from build123d import *

# Parameters (mm, degrees)
SKETCH1_W           = 27.5
SKETCH1_H           = 65
BOSS_EXTRUDE1_DEPTH = 5
SKETCH2_W           = 55
SKETCH2_H           = 130
SKETCH2_W_2         = 45
SKETCH2_H_2         = 120
BOSS_EXTRUDE2_DEPTH = 50.5
SKETCH3_W           = 10
SKETCH3_H           = 10
BOSS_EXTRUDE4_DEPTH = 5
SKETCH4_R           = 2
CUT_EXTRUDE1_DEPTH  = 5
FILLET1_R           = 1
FILLET2_R           = 1
SKETCH6_W           = 38
SKETCH6_H           = 45.3
CUT_EXTRUDE2_DEPTH  = 5
FILLET3_R           = 3
CUT_EXTRUDE3_DEPTH  = 5
FILLET4_R           = 2


with BuildPart() as part:
    # Sketch1 → Boss-Extrude1 (new body)
    with BuildSketch(Plane(origin=(0, 0, 0), x_dir=(1, 0, 0), z_dir=(0, 1, 0))):
        Polygon((27.5, 0), (0, 0), (0, 65), (-27.5, 65), (-27.5, -65), (27.5, -65), align=None)
        with Locations((13.75, 32.5)):
            Rectangle(SKETCH1_W, SKETCH1_H)
    extrude(amount=BOSS_EXTRUDE1_DEPTH)

    # Sketch2 → Boss-Extrude2 (add)
    with BuildSketch(Plane(origin=(0, 5, 0), x_dir=(1, 0, 0), z_dir=(0, 1, 0))):
        Rectangle(SKETCH2_W, SKETCH2_H)
        Rectangle(SKETCH2_W_2, SKETCH2_H_2, mode=Mode.SUBTRACT)
    extrude(amount=BOSS_EXTRUDE2_DEPTH)

    # Sketch3 → Boss-Extrude4 (add)
    with BuildSketch(Plane(origin=(0, 55.5, 0), x_dir=(1, 0, 0), z_dir=(0, 1, 0))):
        with Locations((22.5, 70)):
            Rectangle(SKETCH3_W, SKETCH3_H)
        with Locations((-22.5, -70)):
            Rectangle(SKETCH3_W, SKETCH3_H)
    extrude(amount=-BOSS_EXTRUDE4_DEPTH)

    # Sketch4 → Cut-Extrude1 (cut)
    with BuildSketch(Plane.XZ.offset(-50.5)):
        with Locations(Location((22.5, -70, 0), (0, 0, 270))):
            Circle(SKETCH4_R)
        with Locations(Location((-22.5, 70, 0), (0, 0, 270))):
            Circle(SKETCH4_R)
    extrude(amount=-CUT_EXTRUDE1_DEPTH, mode=Mode.SUBTRACT)

    # Fillet1
    fillet1_edges = [part.edges().sort_by_distance(p)[0] for p in [
        (22.5, 50.5, -68),
    ]]
    fillet(fillet1_edges, radius=FILLET1_R)

    # Fillet2
    fillet2_edges = [part.edges().sort_by_distance(p)[0] for p in [
        (-22.5, 50.5, 72),
    ]]
    fillet(fillet2_edges, radius=FILLET2_R)

    # Sketch6 → Cut-Extrude2 (cut)
    with BuildSketch(Plane.XZ):
        Rectangle(SKETCH6_W, SKETCH6_H)
    extrude(amount=-CUT_EXTRUDE2_DEPTH, mode=Mode.SUBTRACT)

    # Fillet3
    fillet3_edges = [part.edges().sort_by_distance(p)[0] for p in [
        (17.5, 53, -75),
        (27.5, 53, -75),
        (-17.5, 53, 75),
        (-27.5, 53, 75),
    ]]
    fillet(fillet3_edges, radius=FILLET3_R)

    # Sketch8 → Cut-Extrude3 (cut)
    with BuildSketch(Plane(origin=(0, 0, -65), x_dir=(-1, 0, 0), z_dir=(0, 0, -1))):
        Polygon((0, 55.5), (5, 55.5), (5, 45.5), (-5, 45.5), (-5, 55.5), align=None)
    extrude(amount=-CUT_EXTRUDE3_DEPTH, mode=Mode.SUBTRACT)

    # Fillet4
    fillet4_edges = [part.edges().sort_by_distance(p)[0] for p in [
        (-5, 45.5, -62.5),
        (5, 45.5, -62.5),
    ]]
    fillet(fillet4_edges, radius=FILLET4_R)


solid = part.part
The listing builds one solid part. Answer for the finished solid, in the listing's coordinates (mm). A direction names the side the tool comes from. Give positions to 0.01 mm unless a question says otherwise; leave off trailing zeros. Write each loop counter-clockwise with the first axis right and the second up, starting at its lowest first coordinate (ties: lowest second). Pieces come first, ordered by that corner, then holes.
Item 1: Section D-D, the plane z = -4 is taken. Write down the section's boundary in (x, y).
Item 2: Which of the six approach directions +Z, -Z, +X, -X, +Y, -Y give full straight-line access (tool end or side, diameter ignored) to faces 1 (the flat face through (22.5, 30, 1)), 2 (the flat face through (19, 2, 0)), 3 (the flat face through (0, 45.5, -63)), 4 (the flat face through (17.5, 53, -68))?
Item 3: Section C-C, the plane y = 39 is taken. Write down the section's boundary in (x, z), plus the area to 3 significant figures.
Item 4: Section B-B, the plane z = 70 is taken. Write down the section's boundary in (x, y), plus the area to 3 significant figures.
Item 5: Section A-A, the plane x = -14.5 is taken. Write down the section's boundary in (y, z).
Item 6: Flat-ended cylindrical pins translate along their axes: P1, Ø2, axis at x = -2, y = 32.5, coming from the -Z side; P2, Ø4, axis at x = 4, z = -44, coming from the +Y side; P3, Ø1.5, axis at y = 53.5, z = -67.5, coming from the -X side. Find the tip coordinate at first contact, or state that the pin passes through.
Item 7: Find the intervals of material crossed by line 1 along Z through (x, y) = (19, 45); line 2 along X through (y, z) = (54.2, 70); line 3 along Z through (x, y) = (22, 53), in increasing order.
Item 8: Determine the mould class of faces 5 (the cylindrical face through (-18.4, 52.96, 74.14)), 6 (the flat face through (-25, 50.5, 68)), 7 (the flat face through (20, 5, -1)) for opening direction X: released by +X, released by -X, zero draft, split by the parting line, or undercut.
Completed:
1. outline: (-27.5, 0) - (-19, 0) - (-19, 5) - (-22.5, 5) - (-22.5, 55.5) - (-27.5, 55.5) - close; (19, 0) - (27.5, 0) - (27.5, 55.5) - (22.5, 55.5) - (22.5, 5) - (19, 5) - close
2. face 1: +Y
2. face 2: +Y, -Y
2. face 3: -Z, +Y
2. face 4: -Z, -X, +Y, -Y
3. outline: (-27.5, -65) - (27.5, -65) - (27.5, 65) - (-27.5, 65) - close; hole (-22.5, -60) - (22.5, -60) - (22.5, 60) - (-22.5, 60) - close
3. area: 1,750 mm2
4. outline: (-27.5, 50.5) - (-25.5, 50.5) arc R1 ccw to (-24.5, 51.5) - (-24.5, 55.5) - (-27.5, 55.5) - close; (-20.5, 51.5) arc R1 ccw to (-19.5, 50.5) - (-17.5, 50.5) - (-17.5, 55.5) - (-20.5, 55.5) - close
4. area: 29.6 mm2
5. outline: (0, -65) - (55.5, -65) - (55.5, -60) - (5, -60) - (5, -22.65) - (0, -22.65) - close; (0, 22.65) - (5, 22.65) - (5, 60) - (55.5, 60) - (55.5, 65) - (0, 65) - close
6. P1: stops at z = -65
6. P2: stops at y = 5
6. P3: stops at x = 17.5
7. line 1: z = -65 to -60, 60 to 65
7. line 2: x = -27.5 to -24.5, -20.5 to -17.5
7. line 3: z = -75 to -71.94, -68.06 to -60, 60 to 65
8. face 5: released by +X
8. face 6: zero draft
8. face 7: undercut
